```python
from build123d import *

# Parameters (mm, degrees)
F0_R     = 128.5875
F1_DEPTH = 63.5
F2_W     = 44.45
F2_H     = 101.6
F4_R     = 12.7
F5_DEPTH = 63.5
F7_DEPTH = 63.501


with BuildPart() as f1:
    # F0 (on Front) → F1 (new body)
    with BuildSketch(Plane.XZ):
        Circle(F0_R)
    extrude(amount=F1_DEPTH)

    # F2 (on Right) → F3 (revolve, cut)
    with BuildSketch(Plane.YZ):
        with Locations((-31.75, 88.9)):
            Rectangle(F2_W, F2_H)
    revolve(axis=Axis((0, -121.1639214932, 0), (0, 1, 0)), mode=Mode.SUBTRACT)

    # F4 (on face) → F5 (join, through all)
    with BuildSketch(Plane.XZ.offset(63.5)):
        with Locations((0, 116.5098)):
            Circle(F4_R)
        with Locations((-68.4827421875, 94.2584082112)):
            Circle(F4_R)
        with Locations((-110.8074045022, 36.0035082112)):
            Circle(F4_R)
        with Locations((-110.8074045022, -36.0035082112)):
            Circle(F4_R)
        with Locations((-68.4827421875, -94.2584082112)):
            Circle(F4_R)
        with Locations((0, -116.5098)):
            Circle(F4_R)
        with Locations((68.4827421875, -94.2584082112)):
            Circle(F4_R)
        with Locations((110.8074045022, -36.0035082112)):
            Circle(F4_R)
        with Locations((110.8074045022, 36.0035082112)):
            Circle(F4_R)
        with Locations((68.4827421875, 94.2584082112)):
            Circle(F4_R)
    extrude(amount=-F5_DEPTH)

    # F6 (on face) → F7 (cut, through all)
    with BuildSketch(Plane.XZ.offset(63.5)):
        with BuildLine():
            Line((-1.5875, 12.7), (-1.5875, 10.9985226281))
            ThreePointArc((-1.5875, 10.9985226281), (0, -11.1125), (1.5875, 10.9985226281))
            Line((1.5875, 10.9985226281), (1.5875, 12.7))
            Line((1.5875, 12.7), (-1.5875, 12.7))
        make_face()
    extrude(amount=-F7_DEPTH, mode=Mode.SUBTRACT)


solid = f1.part
```
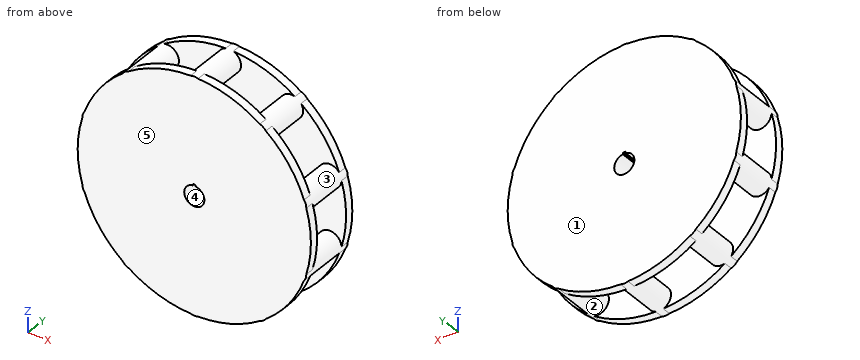
The listing builds one solid part. Answer for the finished solid, in the listing's coordinates (mm). Face numbers are marked on the shaded views. A direction names the side the tool comes from. Coordinates: 2 decimals unless noted, no trailing zeros. Write each loop counter-clockwise with the first axis right and the second up, starting at its lowest first coordinate (ties: lowest second). Pieces come first, ordered by that corner, then holes. Notation, with made-up numbers: M 22.25,80.5 L 63.25,80.5 A3 cw 63.25,84.5 Z; hole C 32,-12.75 d8. An arc over 180 degrees is marked long. Use a Markdown table: item, result. Add a question column.
1. Which of the six approach directions +Z, -Z, +X, -X, +Y, -Y give full straight-line access (tool end or side, diameter ignored) to the marked faces 1 and 2?
2. Straight lines are drawn through the part: line 1 along X through (y, z) = (-26.5, 0); line 2 along Y through (x, z) = (-11, 73) (3 decimals); line 3 along X through (y, z) = (-39, -30). For each, find the intervals that lie inside material, in ascending order. Write a range as [from, to].
3. Section B-B (y = -38) is taken. Count the separate pieces of the cut face and the enclosed holes in it, plus the area to 3 significant figures.
4. For a pull along Y with two mould halves and no side action, classify the marked faces 3, 4 and 5 as +Y half, -Y half, draft (parallel to the pull), parting line (faces both ways), or undercut.
5. Section D-D (z = 27.5) is taken. Give the vertices of the cut face in (x, y) (3 decimals), plus the area to 3 significant figures.
6. Given P1, Ø2, axis at x = 5, y = -21.5, coming from the -Z side; P2, Ø4, axis at y = -12, z = -13, coming from the -X side; P3, Ø1.9, axis at y = -18, z = 11.5, coming from the +X side, each flat-ended and moving along its own axis, determine where each tip first touches the part or whether it passes through.
7. Section A-A (z = 0) is taken. Give the vertices of the cut face in (x, y) (1 decimal), plus the area to 4 significant figures.
8. Section C-C (x = 92) is taken. Give the vertices of the cut face in (y, z) (3 decimals).
Data:
| question | item | result |
|---|---|---|
| 1 | face 1 | +Z, -Z, +X, -X, +Y |
| 1 | face 2 | none |
| 2 | line 1 | x = [-38.1, -11.11], [11.11, 38.1] |
| 2 | line 2 | y = [-63.5, -53.975], [-9.525, 0] |
| 2 | line 3 | x = [-122, -99.62], [-23.49, 23.49], [99.62, 122] |
| 3 | separate pieces | 11 |
| 3 | enclosed holes | 1 |
| 3 | area | 9,230 mm2 |
| 4 | face 3 | undercut |
| 4 | face 4 | draft |
| 4 | face 5 | -Y half |
| 5 | outline | M -125.612,-63.5 L 125.612,-63.5 L 125.612,-53.975 L 120.24,-53.975 L 120.24,-9.525 L 125.612,-9.525 L 125.612,0 L -125.612,0 L -125.612,-9.525 L -120.24,-9.525 L -120.24,-53.975 L -125.612,-53.975 Z; hole M -101.374,-53.975 L -26.37,-53.975 L -26.37,-9.525 L -101.374,-9.525 Z; hole M 26.37,-53.975 L 101.374,-53.975 L 101.374,-9.525 L 26.37,-9.525 Z |
| 5 | area | 8,810 mm2 |
| 6 | P1 | stops at z = -128.56 |
| 6 | P2 | stops at x = -36.48 |
| 6 | P3 | stops at x = 36.61 |
| 7 | outline | M -128.6,-63.5 L -11.1,-63.5 L -11.1,0 L -128.6,0 L -128.6,-9.5 L -38.1,-9.5 L -38.1,-54 L -128.6,-54 Z; M 11.1,-63.5 L 128.6,-63.5 L 128.6,-54 L 38.1,-54 L 38.1,-9.5 L 128.6,-9.5 L 128.6,0 L 11.1,0 Z |
| 7 | area | 6,875 mm2 |
| 8 | outline | M -63.5,-89.837 L -53.975,-89.837 L -53.975,89.837 L -63.5,89.837 Z; M -9.525,-89.837 L 0,-89.837 L 0,89.837 L -9.525,89.837 Z |
